Input: part model. Units: mm. Frame: model coordinates. A direction names the side the tool comes from. Coordinates: 2 decimals unless noted, no trailing zeros. Write each loop counter-clockwise with the first axis right and the second up, starting at its lowest first coordinate (ties: lowest second). Pieces come first, ordered by that corner, then holes. Notation, with made-up numbers: (81.25, 27) - (86.25, 27) arc R23 cw to (86.25, 61) - close; hole circle Ø8 at (42, 50). An arc over 180 degrees is marked (long way). Use CSV: the item, a comma, the result in double quotes.
```python
from build123d import *

# Parameters (mm, degrees)
SKETCH1_W           = 50
SKETCH1_H           = 50
SKETCH1_W_2         = 20
SKETCH1_H_2         = 20
BOSS_EXTRUDE1_DEPTH = 50


with BuildPart() as part:
    # Sketch1 → Boss-Extrude1 (new body)
    with BuildSketch(Plane(origin=(0, 0, 0), x_dir=(1, 0, 0), z_dir=(0, 1, 0))):
        Polygon((-98.419958922, -10.98752745), (-151.112267161, -10.98752745), (-151.112267161, -219.278466068), (-151.112267161, -380.152018312), (-151.112267161, -410.98752745), (-101.112267161, -410.98752745), (-101.112267161, -360.98752745), (-101.112267161, -60.98752745), (198.887732839, -60.98752745), (198.887732839, -360.98752745), (198.887732839, -410.98752745), (248.887732839, -410.98752745), (248.887732839, -380.152018312), (248.887732839, -219.278466068), (248.887732839, -10.98752745), (169.957323972, -10.98752745), align=None)
        with Locations((173.887732839, -385.98752745)):
            Rectangle(SKETCH1_W, SKETCH1_H)
        Polygon((-101.112267161, -360.98752745), (-101.112267161, -410.98752745), (-51.112267161, -410.98752745), (-51.112267161, -360.98752745), (-66.112267161, -360.98752745), (-86.112267161, -360.98752745), align=None)
        with Locations((-76.112267161, -350.98752745)):
            Rectangle(SKETCH1_W_2, SKETCH1_H_2)
        with Locations((173.887732839, -350.98752745)):
            Rectangle(SKETCH1_W_2, SKETCH1_H_2)
    extrude(amount=BOSS_EXTRUDE1_DEPTH)


solid = part.part
```
(1) Reachability of faces 1 (the flat face through (163.888, 25, 351)), 2 (the flat face through (-51.112, 25, 386)), 3 (the flat face through (-11, 50, 47)) from +Z, -Z, +X, -X, +Y, -Y: full face, straight path, thin tool, end or side. Return the list, or none.
Check values:
face 1,"+Y, -Y"
face 2,"+Z, +Y, -Y"
face 3,"+Z, -Z, +X, -X, +Y"
(2) Cut plane C-C on y = 29. Return loops of the section in (x, z).
Check values:
outline,"(-151.11, 10.99) - (248.89, 10.99) - (248.89, 410.99) - (148.89, 410.99) - (148.89, 360.99) - (163.89, 360.99) - (163.89, 340.99) - (183.89, 340.99) - (183.89, 360.99) - (198.89, 360.99) - (198.89, 60.99) - (-101.11, 60.99) - (-101.11, 360.99) - (-86.11, 360.99) - (-86.11, 340.99) - (-66.11, 340.99) - (-66.11, 360.99) - (-51.11, 360.99) - (-51.11, 410.99) - (-151.11, 410.99) - close"
(3) Pin query (flat end, axial travel): pin 1 Ø6 at (x, y) = (71, 24) entering from +Z. Return the tip coordinate at first contact, or that it passes through.
Check values:
pin 1,"z = 60.99"
(4) Cut plane D-D on x = 87.5. Return loops of the section in (y, z).
Check values:
outline,"(0, 10.99) - (50, 10.99) - (50, 60.99) - (0, 60.99) - close"
(5) Draft query along Z for faces 4 (the flat face through (156, 25, 360.988)), 5 (the flat face through (-151.112, 25, 208)), 6 (the flat face through (52, 25, 10.988)). Return one class per face: pulls with the +Z half, pulls with the -Z half, needs draft (parallel to the pull), parting line crosses it, or undercut.
Check values:
face 4,"undercut"
face 5,"needs draft"
face 6,"pulls with the -Z half"
(6) Cut plane B-B on z = 366. Return loops of the section in (x, y), and give its area (3 significant figures).
Check values:
outline,"(-151.11, 0) - (-51.11, 0) - (-51.11, 50) - (-151.11, 50) - close; (148.89, 0) - (248.89, 0) - (248.89, 50) - (148.89, 50) - close"
area,"10,000 mm^2"
(7) Ray query, probe 1 along X at (y, z) = (4.5, 112); probe 2 along Z at (x, y) = (195, 29); probe 3 along Z at (x, y) = (141, 35). Return the intervals inside material, ascending. Write a range as from..to.
Check values:
probe 1,"-151.11..-101.11, 198.89..248.89"
probe 2,"10.99..60.99, 360.99..410.99"
probe 3,"10.99..60.99"
(8) Cut plane A-A on x = -74. Return loops of the section in (y, z), and give its area (3 significant figures).
Check values:
outline,"(0, 10.99) - (50, 10.99) - (50, 60.99) - (0, 60.99) - close; (0, 340.99) - (50, 340.99) - (50, 410.99) - (0, 410.99) - close"
area,"6,000 mm^2"
